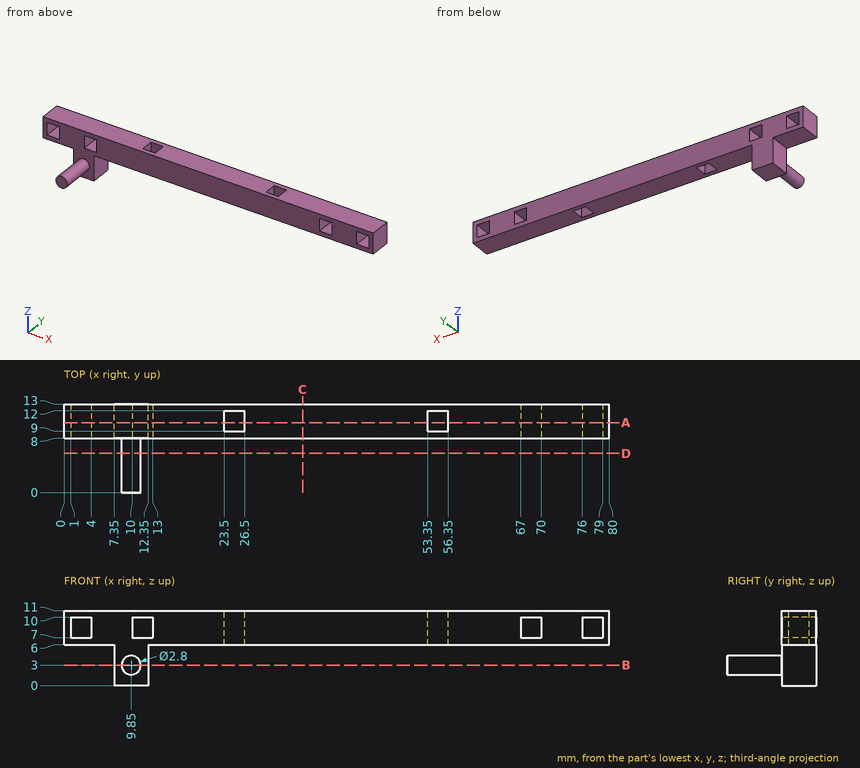
Input: dimensioned drawing with shaded views. Units: mm. Origin: part minimum x, y, z. Coordinates: 2 decimals unless noted, no trailing zeros. Loops run counter-clockwise (first coordinate to the right, second up) from the corner with the lowest first, then second, coordinate; pieces in that order, holes last.
Q1. Section A-A, the plane y = 10.25. Give the number of separate pieces and of enclosed holes in the cut face, and give its area (3 significant figures).
Results are:
separate pieces: 3
enclosed holes: 4
area: 364 mm2
Q2. Section B-B, the plane z = 3. Return the cut outline in (x, y).
Results are:
outline: (7.35, 8) - (8.45, 8) - (8.45, 0) - (11.25, 0) - (11.25, 8) - (12.35, 8) - (12.35, 13) - (7.35, 13) - close
Q3. Section D-D, the plane y = 5.75. Return the cut outline in (x, z).
Results are:
outline: circle Ø2.8 at (9.85, 3)
Q4. Contact query for flat-ended pins moving along their axis: pin 1 (4 mm diameter, centred on y = 10, z = 3, fed in from +X); pin 2 (1 mm diameter, centred on x = 16, y = 7, fed in from -Z); pin 3 (2 mm diameter, centred on y = 9.5, z = 1.5, fed in from -X); pin 4 (1 mm diameter, centred on x = 24, z = 6.5, fed in from -Y). Output: stop coordinate, or through.
Results are:
pin 1: stops at x = 12.35
pin 2: passes through
pin 3: stops at x = 7.35
pin 4: stops at y = 8
Q5. Section C-C, the plane x = 35. Return the cut outline in (y, z).
Results are:
outline: (8, 6) - (13, 6) - (13, 11) - (8, 11) - close
Q6. Line query: line 1 along X through (y, z) = (11, 6.5); line 2 along Y through (x, z) = (28, 7.75); line 3 along X through (y, z) = (9.25, 1.5). Output: solid intervals per line, ascending.
Results are:
line 1: x = 0 to 23.5, 26.5 to 53.35, 56.35 to 80
line 2: y = 8 to 13
line 3: x = 7.35 to 12.35
